from build123d import *

# Parameters (mm, degrees)
F0_W     = 228.6
F0_H     = 228.6
F0_W_2   = 63.5
F0_H_2   = 63.5
F1_DEPTH = 5.08
F2_W     = 38.1
F2_H     = 38.1
F3_DEPTH = 25.4
F4_R     = 7.62
F5_W     = 38.1
F5_H     = 38.1
F6_DEPTH = 25.4
F7_R     = 5.08
F8_R     = 5.08


with BuildPart() as f1:
    # F0 (on Top) → F1 (new body)
    with BuildSketch(Plane.XY):
        Rectangle(F0_W, F0_H)
        Rectangle(F0_W_2, F0_H_2, mode=Mode.SUBTRACT)
    extrude(amount=F1_DEPTH)

    # F2 (on face) → F3 (cut)
    with BuildSketch(Plane.XY.offset(5.08)):
        with Locations((-63.5, 63.5)):
            Rectangle(F2_W, F2_H)
    extrude(amount=-F3_DEPTH, mode=Mode.SUBTRACT)

    # F4
    f4_edges = [f1.edges().sort_by_distance(p)[0] for p in [
        (-82.55, 82.55, 2.54),
        (-44.45, 82.55, 2.54),
        (-44.45, 44.45, 2.54),
        (-82.55, 44.45, 2.54),
    ]]
    fillet(f4_edges, radius=F4_R)

    # F5 (on face) → F6 (cut)
    with BuildSketch(Plane.XY.offset(5.08)):
        with Locations((-63.5, 0)):
            Rectangle(F5_W, F5_H)
        with Locations((0, 63.5)):
            Rectangle(F5_W, F5_H)
        with Locations((63.5, 63.5)):
            Rectangle(F5_W, F5_H)
        with Locations((63.5, 0)):
            Rectangle(F5_W, F5_H)
        with Locations((63.5, -63.5)):
            Rectangle(F5_W, F5_H)
        with Locations((0, -63.5)):
            Rectangle(F5_W, F5_H)
        with Locations((-63.5, -63.5)):
            Rectangle(F5_W, F5_H)
    extrude(amount=-F6_DEPTH, mode=Mode.SUBTRACT)

    # F7
    f7_edges = [f1.edges().sort_by_distance(p)[0] for p in [
        (-82.55, 19.05, 2.54),
        (-82.55, -44.45, 2.54),
        (-31.75, 31.75, 2.54),
        (-19.05, 82.55, 2.54),
        (44.45, 19.05, 2.54),
        (44.45, 82.55, 2.54),
        (44.45, -44.45, 2.54),
        (-19.05, -44.45, 2.54),
        (82.55, 82.55, 2.54),
        (82.55, 19.05, 2.54),
        (82.55, -44.45, 2.54),
        (19.05, -44.45, 2.54),
        (31.75, 31.75, 2.54),
        (-44.45, -44.45, 2.54),
        (-44.45, 19.05, 2.54),
        (19.05, 82.55, 2.54),
        (19.05, 44.45, 2.54),
        (82.55, -19.05, 2.54),
        (82.55, -82.55, 2.54),
        (19.05, -82.55, 2.54),
        (-44.45, -82.55, 2.54),
        (-44.45, -19.05, 2.54),
        (31.75, -31.75, 2.54),
        (-82.55, -82.55, 2.54),
        (-19.05, -82.55, 2.54),
        (44.45, -82.55, 2.54),
        (44.45, -19.05, 2.54),
        (44.45, 44.45, 2.54),
        (-19.05, 44.45, 2.54),
        (82.55, 44.45, 2.54),
    ]]
    fillet(f7_edges, radius=F7_R)

    # F8
    f8_edges = [f1.edges().sort_by_distance(p)[0] for p in [
        (-31.75, -31.75, 2.54),
    ]]
    fillet(f8_edges, radius=F8_R)


solid = f1.part
Input: part model. Units: mm. Frame: model coordinates. Give positions to 0.01 mm unless a question says otherwise; leave off trailing zeros. Order: outer loops, then holes, each group sorted by start corner. A loop starts at its lowest first (then second) coordinate and runs counter-clockwise, first axis right, second up.
Q1. Section C-C on z = 3.45. State how many separate pieces and enclosed holes the cut face has, and give its area (3 significant figures).
Checked values:
separate pieces: 1
enclosed holes: 9
area: 36,800 mm2
Q2. Section A-A on y = 68. Output: boundary loops of the cut face in (x, z).
Checked values:
outline: (-114.3, 0) - (-82.55, 0) - (-82.55, 5.08) - (-114.3, 5.08) - close; (-44.45, 0) - (-19.05, 0) - (-19.05, 5.08) - (-44.45, 5.08) - close; (19.05, 0) - (44.45, 0) - (44.45, 5.08) - (19.05, 5.08) - close; (82.55, 0) - (114.3, 0) - (114.3, 5.08) - (82.55, 5.08) - close
Q3. Draft query along Y for faces 1 (the flat face through (-64, -44.45, 3)), 2 (the flat face through (-114.3, -2, 3)). Return one class per face: +Y half, -Y half, draft (parallel to the pull), parting line (faces both ways), or undercut.
Checked values:
face 1: undercut
face 2: draft
Q4. Ray query, probe 1 along Y at (x, z) = (2, 1.8); probe 2 along Y at (x, z) = (75, 0.6). Return the intervals inside material, ascending.
Checked values:
probe 1: y = -114.3 to -82.55, -44.45 to -31.75, 31.75 to 44.45, 82.55 to 114.3
probe 2: y = -114.3 to -82.55, -44.45 to -19.05, 19.05 to 44.45, 82.55 to 114.3
